from build123d import *

# Parameters (mm, degrees)
BOSS_EXTRUDE1_DEPTH      = 10
SKETCH2_W                = 23
SKETCH2_H                = 23
CUT_EXTRUDE1_DEPTH       = 3
CUT_EXTRUDE2_DEPTH       = 108.15565003
CUT_EXTRUDE2_DEPTH_BACK  = 108.15565003
SKETCH3_R                = 1.5
CUT_EXTRUDE3_DEPTH       = 108.393357957
CUT_EXTRUDE3_DEPTH_BACK  = 3
SKETCH4_W                = 20.26
SKETCH4_H                = 15.56
CUT_EXTRUDE4_DEPTH       = 108.15565003
CUT_EXTRUDE4_DEPTH_BACK  = 108.15565003
SKETCH5_R                = 1.425
CUT_EXTRUDE6_DEPTH       = 108.393357957
CUT_EXTRUDE6_DEPTH_BACK  = 108.393357957
FILLET1_R                = 5
SKETCH8_W                = 20.26
SKETCH8_H                = 3
CUT_EXTRUDE8_DEPTH       = 28.72
CHAMFER1_SIZE            = 1.37
SKETCH9_R                = 1.65
CUT_EXTRUDE9_DEPTH       = 108.393357957
SKETCH10_R               = 3
CUT_EXTRUDE10_DEPTH      = 5
BOSS_EXTRUDE2_DEPTH      = 2.5
BOSS_EXTRUDE2_DEPTH_BACK = 7
SKETCH12_R               = 1.75
SKETCH12_R_2             = 1.425
CHAMFER2_SIZE            = 2
CHAMFER3_SIZE            = 1.25


# Some blends are built 0.0001 mm under size
with BuildPart() as part:
    # Sketch1 → Boss-Extrude1 (new body)
    with BuildSketch(Plane.XY):
        Polygon((0, -80.829037687), (70, 40.414518843), (-70, 40.414518843), align=None)
    extrude(amount=BOSS_EXTRUDE1_DEPTH)

    # Sketch2 → Cut-Extrude1 (cut)
    with BuildSketch(Plane(origin=(0, 0, 0), x_dir=(-1, 0, 0), z_dir=(0, 0, -1))):
        Rectangle(SKETCH2_W, SKETCH2_H)
    extrude(amount=-CUT_EXTRUDE1_DEPTH, mode=Mode.SUBTRACT)

    # Sketch3 → Cut-Extrude2 (cut, two sides: drawn at the far end of the back side and taken through both)
    with BuildSketch(Plane(origin=(0, 0, 3), x_dir=(-1, 0, 0), z_dir=(0, 0, -1)).offset(-CUT_EXTRUDE2_DEPTH_BACK)):
        with Locations((-8, 8)):
            Circle(SKETCH3_R)
        with Locations((8, 8)):
            Circle(SKETCH3_R)
        with Locations((8, -8)):
            Circle(SKETCH3_R)
        with Locations((-8, -8)):
            Circle(SKETCH3_R)
    extrude(amount=CUT_EXTRUDE2_DEPTH + CUT_EXTRUDE2_DEPTH_BACK, mode=Mode.SUBTRACT)

    # Sketch4 → Cut-Extrude3 (cut, two sides: drawn at the far end of the back side and taken through both)
    with BuildSketch(Plane(origin=(0, 0, 0), x_dir=(-1, 0, 0), z_dir=(0, 0, -1)).offset(-CUT_EXTRUDE3_DEPTH_BACK)):
        with Locations((0, 25)):
            Rectangle(SKETCH4_W, SKETCH4_H)
    extrude(amount=CUT_EXTRUDE3_DEPTH + CUT_EXTRUDE3_DEPTH_BACK, mode=Mode.SUBTRACT)

    # Sketch5 → Cut-Extrude4 (cut, two sides: drawn at the far end of the back side and taken through both)
    with BuildSketch(Plane(origin=(0, 0, 3), x_dir=(-1, 0, 0), z_dir=(0, 0, -1)).offset(-CUT_EXTRUDE4_DEPTH_BACK)):
        with Locations((-7.53, 30.14)):
            Circle(SKETCH5_R)
        with Locations((7.53, 30.14)):
            Circle(SKETCH5_R)
    extrude(amount=CUT_EXTRUDE4_DEPTH + CUT_EXTRUDE4_DEPTH_BACK, mode=Mode.SUBTRACT)

    # Sketch6 → Cut-Extrude6 (cut, two sides: drawn at the far end of the back side and taken through both)
    with BuildSketch(Plane(origin=(0, 0, 0), x_dir=(-1, 0, 0), z_dir=(0, 0, -1)).offset(-CUT_EXTRUDE6_DEPTH_BACK)):
        Polygon((-13.5, 13.5), (-13.5, 35.414518843), (-61.339745962, 35.414518843), (-48.687392609, 13.5), align=None)
        Polygon((13.5, 13.5), (48.687392609, 13.5), (61.339745962, 35.414518843), (13.5, 35.414518843), align=None)
        Polygon((-13.5, -13.5), (-33.098935341, -13.5), (0, -70.829037687), (33.098935341, -13.5), (13.5, -13.5), align=None)
    extrude(amount=CUT_EXTRUDE6_DEPTH + CUT_EXTRUDE6_DEPTH_BACK, mode=Mode.SUBTRACT)

    # Fillet1
    fillet1_edges = [part.edges().sort_by_distance(p)[0] for p in [
        (13.5, 35.414518843, 5),
        (13.5, 13.5, 5),
        (48.687392609, 13.5, 5),
        (61.339745962, 35.414518843, 5),
        (33.098935341, -13.5, 5),
        (-33.098935341, -13.5, 5),
        (0, -70.829037687, 5),
        (-48.687392609, 13.5, 5),
        (-13.5, 13.5, 5),
        (-13.5, 35.414518843, 5),
        (-61.339745962, 35.414518843, 5),
    ]]
    fillet(fillet1_edges, radius=FILLET1_R)

    # Sketch8 → Cut-Extrude8 (cut)
    with BuildSketch(Plane(origin=(0, 17.22, 0), x_dir=(1, 0, 0), z_dir=(0, 1, 0))):
        with Locations((0, -1.5)):
            Rectangle(SKETCH8_W, SKETCH8_H)
    extrude(amount=-CUT_EXTRUDE8_DEPTH, mode=Mode.SUBTRACT)

    # Chamfer1
    chamfer1_edges = [part.edges().sort_by_distance(p)[0] for p in [
        (10.13, 11.5, 1.5),
        (-10.13, 11.5, 1.5),
    ]]
    chamfer(chamfer1_edges, length=CHAMFER1_SIZE - 0.0001)  # a hair under: the kernel refuses the full size

    # Sketch9 → Cut-Extrude9 (cut, through all)
    with BuildSketch(Plane(origin=(0, 0, 0), x_dir=(-1, 0, 0), z_dir=(0, 0, -1))):
        with Locations((-62.5, 36.084391824)):
            Circle(SKETCH9_R)
        with Locations((62.5, 36.084391824)):
            Circle(SKETCH9_R)
        with Locations((0, -72.168783649)):
            Circle(SKETCH9_R)
    extrude(amount=-CUT_EXTRUDE9_DEPTH, mode=Mode.SUBTRACT)

    # Sketch10 → Cut-Extrude10 (cut)
    with BuildSketch(Plane(origin=(0, 0, 10), x_dir=(-1, 0, 0), z_dir=(0, 0, -1))):
        with Locations(Location((-62.5, 36.084391824, 0), (0, 0, 180))):
            Circle(SKETCH10_R)
        with Locations(Location((62.5, 36.084391824, 0), (0, 0, 180))):
            Circle(SKETCH10_R)
        with Locations(Location((0, -72.168783649, 0), (0, 0, 180))):
            Circle(SKETCH10_R)
    extrude(amount=CUT_EXTRUDE10_DEPTH, mode=Mode.SUBTRACT)

    # Sketch12 → Boss-Extrude2 (add, two sides: drawn at the far end of the back side and taken through both)
    with BuildSketch(Plane(origin=(0, 0, 3), x_dir=(-1, 0, 0), z_dir=(0, 0, -1)).offset(-BOSS_EXTRUDE2_DEPTH_BACK)):
        with Locations((-8, 8)):
            Circle(SKETCH12_R)
        with Locations((8, 8)):
            Circle(SKETCH12_R)
        with Locations((8, -8)):
            Circle(SKETCH12_R)
        with Locations((-8, -8)):
            Circle(SKETCH12_R)
        with Locations((-7.53, 30.14)):
            Circle(SKETCH12_R_2)
        with Locations((7.53, 30.14)):
            Circle(SKETCH12_R_2)
    extrude(amount=BOSS_EXTRUDE2_DEPTH + BOSS_EXTRUDE2_DEPTH_BACK)

    # Chamfer2
    # the kernel refuses this chamfer: 2 mm, written as the material it takes off along each edge
    with BuildSketch(Plane(origin=(62.5, 36.084391824, 5), x_dir=(-1, 0, 0), z_dir=(0, -1, 0))) as chamfer2_piece_1_section:
        Polygon((1.65, CHAMFER2_SIZE), (1.65 + CHAMFER2_SIZE, 0), (1.65, 0), align=None)
    chamfer2_piece_1 = revolve(axis=Axis((62.5, 36.084391824, 5), (0, 0, -1)), mode=Mode.PRIVATE)
    chamfer2_piece_1 = chamfer2_piece_1 & Plane(origin=(62.5, 36.084391824, 3.667830139), x_dir=(1, 0, 0), z_dir=(0, 0, 1)) * Cylinder(3, 15, mode=Mode.PRIVATE)
    add(chamfer2_piece_1, mode=Mode.SUBTRACT)
    with BuildSketch(Plane(origin=(-62.5, 36.084391824, 5), x_dir=(-1, 0, 0), z_dir=(0, -1, 0))) as chamfer2_piece_2_section:
        Polygon((1.65, CHAMFER2_SIZE), (1.65 + CHAMFER2_SIZE, 0), (1.65, 0), align=None)
    chamfer2_piece_2 = revolve(axis=Axis((-62.5, 36.084391824, 5), (0, 0, -1)), mode=Mode.PRIVATE)
    chamfer2_piece_2 = chamfer2_piece_2 & Plane(origin=(-62.5, 36.084391824, 3.667830139), x_dir=(1, 0, 0), z_dir=(0, 0, 1)) * Cylinder(3, 15, mode=Mode.PRIVATE)
    add(chamfer2_piece_2, mode=Mode.SUBTRACT)
    with BuildSketch(Plane(origin=(0, -72.168783649, 5), x_dir=(-1, 0, 0), z_dir=(0, -1, 0))) as chamfer2_piece_3_section:
        Polygon((1.65, CHAMFER2_SIZE), (1.65 + CHAMFER2_SIZE, 0), (1.65, 0), align=None)
    chamfer2_piece_3 = revolve(axis=Axis((0, -72.168783649, 5), (0, 0, -1)), mode=Mode.PRIVATE)
    chamfer2_piece_3 = chamfer2_piece_3 & Plane(origin=(0, -72.168783649, 3.667830139), x_dir=(1, 0, 0), z_dir=(0, 0, 1)) * Cylinder(3, 15, mode=Mode.PRIVATE)
    add(chamfer2_piece_3, mode=Mode.SUBTRACT)

    # Chamfer3
    chamfer3_edges = [part.edges().sort_by_distance(p)[0] for p in [
        (9.75, 8, 0.5),
        (-6.25, 8, 0.5),
        (-6.25, -8, 0.5),
        (9.75, -8, 0.5),
        (8.955, 30.14, 0.5),
        (-6.105, 30.14, 0.5),
    ]]
    chamfer(chamfer3_edges, length=CHAMFER3_SIZE)


solid = part.part
Here's how the part is built. I have some questions about the finished solid (model axes, mm). A direction names the side the tool comes from. Round coordinates to 2 decimals unless told otherwise and drop trailing zeros. Loops run counter-clockwise (first coordinate to the right, second up) from the corner with the lowest first, then second, coordinate; pieces in that order, holes last.
1. Which directions (+Z, -Z, +X, -X, +Y, -Y) give clear straight access to the entire face, cutting with the end or side of a thin tool? Please do faces 4 (the face through (-7.344, 31.553, 2.384)), 5 (the face through (-28.732, -15.937, 4.93)), 6 (the face through (1, 40.415, 5)).
Answer list:
face 4: -Z
face 5: +Z, -Z
face 6: +Z, -Z, +X, -X, +Y
2. If we section it at A-A on x = 44: Write out the boundary of the cut face in (y, z).
Answer list:
outline: (-4.62, 0) - (13.5, 0) - (13.5, 10) - (-4.62, 10) - close; (35.41, 0) - (40.41, 0) - (40.41, 10) - (35.41, 10) - close
3. For P1, Ø3, axis at x = 62.5, y = 36.08, coming from the -Z side; P2, Ø0.8, axis at x = -8, y = -8, coming from the -Z side; P3, Ø4, axis at y = -43, z = 7.5, coming from the +X side; P4, Ø0.9, axis at y = 1, z = 1.5, coming from the -X side, each with a flat end and sliding along its axis, tell me the tip position at first contact or that it passes through.
Answer list:
P1: passes through
P2: stops at z = 0.5
P3: stops at x = 23
P4: stops at x = -47.5
4. If I drill on line 1 along Y through (x, z) = (0, 1.75); line 2 along Y through (x, z) = (0, 4.55); line 3 along Y through (x, z) = (6.5, 1), over which ranges is the centre line in solid material (lowest first)?
Answer list:
line 1: y = -80.83 to -73.82, -70.52 to -65.83, -13.5 to -11.5, 32.78 to 40.41
line 2: y = -80.83 to -75.17, -69.17 to -65.83, -13.5 to 40.41
line 3: y = -69.57 to -59.57, -13.5 to -11.5, 32.78 to 40.41
5. If we section it at D-D on y = -23: Write out the boundary of the cut face in (x, z).
Answer list:
outline: (-33.39, 0) - (-27.61, 0) - (-27.61, 10) - (-33.39, 10) - close; (27.61, 0) - (33.39, 0) - (33.39, 10) - (27.61, 10) - close
6. If we section it at C-C on x = 20.5: Write out the boundary of the cut face in (y, z).
Answer list:
outline: (-45.32, 0) - (-35.32, 0) - (-35.32, 10) - (-45.32, 10) - close; (-13.5, 0) - (13.5, 0) - (13.5, 10) - (-13.5, 10) - close; (35.41, 0) - (40.41, 0) - (40.41, 10) - (35.41, 10) - close
7. If we section it at B-B on z = 8.5: Write out the boundary of the cut face in (x, y).
Answer list:
outline: (-70, 40.41) - (0, -80.83) - (70, 40.41) - close; hole circle Ø6 at (-62.5, 36.08); hole (-57.01, 27.91) - (-50.13, 16) arc R5 ccw to (-45.8, 13.5) - (-18.5, 13.5) arc R5 ccw to (-13.5, 18.5) - (-13.5, 30.41) arc R5 ccw to (-18.5, 35.41) - (-52.68, 35.41) arc R5 ccw to start; hole (-28.77, -21) - (-4.33, -63.33) arc R5 ccw to (4.33, -63.33) - (28.77, -21) arc R5 ccw to (24.44, -13.5) - (-24.44, -13.5) arc R5 ccw to start; hole circle Ø6 at (0, -72.17); hole (13.5, 18.5) arc R5 ccw to (18.5, 13.5) - (45.8, 13.5) arc R5 ccw to (50.13, 16) - (57.01, 27.91) arc R5 ccw to (52.68, 35.41) - (18.5, 35.41) arc R5 ccw to (13.5, 30.41) - close; hole circle Ø6 at (62.5, 36.08)
8. We'd pull the mould along X, two halves only. Please class faces 1 (the face through (-36, 35.415, 5)), 2 (the face through (34.51, -21.056, 4.93)), 3 (the face through (-16, 7, 0)): +X half, -X half, draft (parallel to the pull), parting line (faces both ways), or undercut.
Answer list:
face 1: undercut
face 2: +X half
face 3: draft
